Part model, mm, in its own coordinate system. Coordinates: 2 decimals unless noted, no trailing zeros. Loops run counter-clockwise (first coordinate to the right, second up) from the corner with the lowest first, then second, coordinate; pieces in that order, holes last. Notation, with made-up numbers: (58.25, 34.5) -> (103.25, 34.5) arc R14 cw to (103.25, 40.5) -> close; hole circle Ø5 at (13.25, 19). An arc over 180 degrees is marked (long way). Use one line per item in the form item = value. Start each with the question number.
(1) Drill centre lines: L1, parallel to Y at x = 1.85, z = 33.5; L2, parallel to Y at x = 1.8, z = 22.5; L3, parallel to Z at x = 5.6, y = 15 (3 decimals). Where is each one in solid material? Low to high. Write a range as [from, to].
(2) Band-saw the part on C-C on x = 2.85. Count the separate pieces of the cut face and the enclosed holes in it, then the cut area to 3 significant figures.
(3) Band-saw the part on B-B on y = 0.5. Give the cut face in (x, z).
(4) Band-saw the part on D-D on z = 2.5. Give the cut face in (x, y).
(5) Band-saw the part on A-A on z = -23. Give the cut face in (x, y).
(6) Pin check, flat tips, straight feed: P1, Ø3, axis at x = 3.5, z = -54, coming from the +Y side; P2, Ø5, axis at y = 79, z = -53.29, coming from the -X side; P3, Ø10, axis at y = 1.5, z = -10, coming from the +X side; P4, Ø1.8, axis at x = 2, y = -121.5, coming from the -Z side. Stop position of each tip, or through.
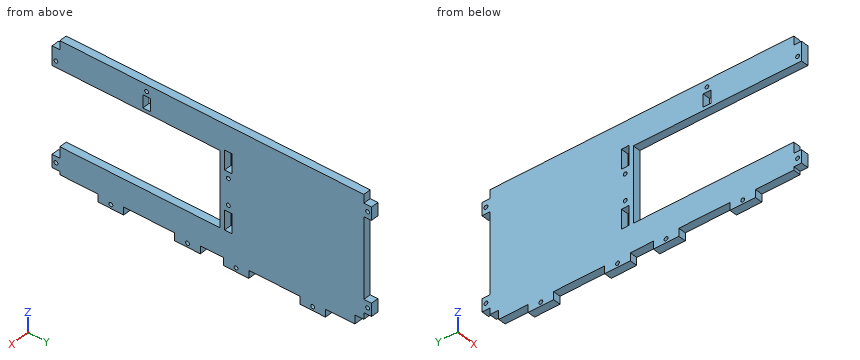
```python
from build123d import *

# Parameters (mm, degrees)
ESQUISSE1_W             = 100.58
ESQUISSE1_H             = 238
ESQUISSE1_W_2           = 10
ESQUISSE1_H_2           = 6
ESQUISSE1_W_3           = 15
BOSS_EXTRU_1_DEPTH      = 6
ESQUISSE3_W             = 20
ESQUISSE3_H             = 6
ESQUISSE3_W_2           = 10
ESQUISSE3_W_3           = 6
ESQUISSE3_H_2           = 20
BOSS_EXTRU_5_DEPTH      = 6
ESQUISSE6_W             = 58
ESQUISSE6_H             = 131.59
ENL_V_MAT_EXTRU_2_DEPTH = 6
ESQUISSE7_W             = 6.88
ESQUISSE7_H             = 7
ENL_V_MAT_EXTRU_3_DEPTH = 6
ESQUISSE8_R             = 1.5
ENL_V_MAT_EXTRU_4_DEPTH = 6


with BuildPart() as part:
    # Esquisse1 → Boss.-Extru.1 (new body)
    with BuildSketch(Plane(origin=(0, 0, 0), x_dir=(0, 0, -1), z_dir=(1, 0, 0))):
        Rectangle(ESQUISSE1_W, ESQUISSE1_H)
        with Locations((-36.29, -51)):
            Rectangle(ESQUISSE1_W_2, ESQUISSE1_H_2, mode=Mode.SUBTRACT)
        with Locations((-23.295, 13)):
            Rectangle(ESQUISSE1_W_3, ESQUISSE1_H_2, mode=Mode.SUBTRACT)
        with Locations((21.705, 13)):
            Rectangle(ESQUISSE1_W_3, ESQUISSE1_H_2, mode=Mode.SUBTRACT)
    extrude(amount=BOSS_EXTRU_1_DEPTH)

    # Esquisse3 → Boss.-Extru.5 (add)
    with BuildSketch(Plane(origin=(6, 0, 0), x_dir=(0, 0, -1), z_dir=(1, 0, 0))):
        with Locations((-33.5, -122)):
            Rectangle(ESQUISSE3_W, ESQUISSE3_H)
        with Locations((42.79, -122)):
            Rectangle(ESQUISSE3_W_2, ESQUISSE3_H)
        with Locations((53.29, 19)):
            Rectangle(ESQUISSE3_W_3, ESQUISSE3_H_2)
        with Locations((53.29, 79)):
            Rectangle(ESQUISSE3_W_3, ESQUISSE3_H_2)
        with Locations((53.29, -79)):
            Rectangle(ESQUISSE3_W_3, ESQUISSE3_H_2)
        with Locations((53.29, -19)):
            Rectangle(ESQUISSE3_W_3, ESQUISSE3_H_2)
        with Locations((33.41, 122)):
            Rectangle(ESQUISSE3_W_2, ESQUISSE3_H)
        with Locations((-38.71, 122)):
            Rectangle(ESQUISSE3_W_2, ESQUISSE3_H)
    extrude(amount=-BOSS_EXTRU_5_DEPTH)

    # Esquisse6 → Enlèv. mat.-Extru.2 (cut)
    with BuildSketch(Plane(origin=(6, 0, 0), x_dir=(0, 0, -1), z_dir=(1, 0, 0))):
        with Locations((0.29, -59.205)):
            Rectangle(ESQUISSE6_W, ESQUISSE6_H)
    extrude(amount=-ENL_V_MAT_EXTRU_2_DEPTH, mode=Mode.SUBTRACT)

    # Esquisse7 → Enlèv. mat.-Extru.3 (cut)
    with BuildSketch(Plane.ZY):
        with Locations((-46.85, 115.5)):
            Rectangle(ESQUISSE7_W, ESQUISSE7_H)
    extrude(amount=-ENL_V_MAT_EXTRU_3_DEPTH, mode=Mode.SUBTRACT)

    # Esquisse8 → Enlèv. mat.-Extru.4 (cut)
    with BuildSketch(Plane.ZY):
        with Locations((-9.205, 13)):
            Circle(ESQUISSE8_R)
        with Locations((10.795, 13)):
            Circle(ESQUISSE8_R)
        with Locations((45.08, -51)):
            Circle(ESQUISSE8_R)
        with Locations((38.71, 122)):
            Circle(ESQUISSE8_R)
        with Locations((-33.41, 122)):
            Circle(ESQUISSE8_R)
        with Locations((33.5, -122)):
            Circle(ESQUISSE8_R)
        with Locations((-53.29, 79)):
            Circle(ESQUISSE8_R)
        with Locations((-42.79, -122)):
            Circle(ESQUISSE8_R)
        with Locations((-53.29, 19)):
            Circle(ESQUISSE8_R)
        with Locations((-53.29, -79)):
            Circle(ESQUISSE8_R)
        with Locations((-53.29, -19)):
            Circle(ESQUISSE8_R)
    extrude(amount=-ENL_V_MAT_EXTRU_4_DEPTH, mode=Mode.SUBTRACT)


solid = part.part
```
A:
q1.L1 = [-125, -123.5], [-120.5, -54], [-48, 119]
q1.L2 = [6.59, 10], [16, 119]
q1.L3 = [-56.29, -29.205], [-14.205, 15.795], [30.795, 50.29]
q2.separate_pieces = 1
q2.enclosed_holes = 14
q2.area = 17,000 mm²
q3.outline = (0, -50.29) -> (6, -50.29) -> (6, -29.29) -> (0, -29.29) -> close; (0, 28.71) -> (6, 28.71) -> (6, 50.29) -> (0, 50.29) -> close
q4.outline = (0, 6.59) -> (6, 6.59) -> (6, 119) -> (0, 119) -> close
q5.outline = (0, 6.59) -> (6, 6.59) -> (6, 10) -> (0, 10) -> close; (0, 16) -> (6, 16) -> (6, 119) -> (0, 119) -> close
q6.P1 = 89
q6.P2 = 0
q6.P3 = through
q6.P4 = -47.79
